Design review of the part built by this model. Coordinates are the model's own, in mm. Round coordinates to 2 decimals unless told otherwise and drop trailing zeros. Order: outer loops, then holes, each group sorted by start corner. A loop starts at its lowest first (then second) coordinate and runs counter-clockwise, first axis right, second up.
from build123d import *

# Parameters (mm, degrees)
SZKIC1_R                    = 5
DODANIE_WYCI_GNI_CIE1_DEPTH = 2


with BuildPart() as part:
    # Szkic1 → Dodanie-wyciągnięcie1 (new body)
    with BuildSketch(Plane.XY):
        Polygon((0, 0), (0, -100), (-100, 0), align=None)
        with Locations((-50, -13)):
            Circle(SZKIC1_R, mode=Mode.SUBTRACT)
        with Locations((-13, -50)):
            Circle(SZKIC1_R, mode=Mode.SUBTRACT)
    extrude(amount=DODANIE_WYCI_GNI_CIE1_DEPTH)


solid = part.part
1) Take a section at D-D on x = -29. Give the boundary of the cut face in (y, z).
Results:
outline: (-71, 0) - (0, 0) - (0, 2) - (-71, 2) - close
2) Take a section at C-C on z = 1.6. Give the boundary of the cut face in (x, y).
Results:
outline: (-100, 0) - (0, -100) - (0, 0) - close; hole circle Ø10 at (-50, -13); hole circle Ø10 at (-13, -50)
3) The part is to be moulded in two halves that separate along X. For faces 1 (the face through (-49, -51, 1)), 2 (the face through (-55, -13, 1)), 3 (the face through (-38, -38, 0)), say which applies: released by +X, released by -X, zero draft, split by the parting line, or undercut.
Results:
face 1: released by -X
face 2: undercut
face 3: zero draft
4) To check wall thickness, follow line 1 along Y through (x, z) = (-13, 1.2); line 2 along Y through (x, z) = (-48.5, 1.45); line 3 along Y through (x, z) = (-82, 0.4). State the ranges of each line that lie inside material, in increasing order.
Results:
line 1: y = -87 to -55, -45 to 0
line 2: y = -51.5 to -17.77, -8.23 to 0
line 3: y = -18 to 0
5) Take a section at A-A on y = -50. Give the boundary of the cut face in (x, z).
Results:
outline: (-50, 0) - (-18, 0) - (-18, 2) - (-50, 2) - close; (-8, 0) - (0, 0) - (0, 2) - (-8, 2) - close
